The listing builds one solid part. Answer for the finished solid, in the listing's coordinates (mm). Face numbers are marked on the shaded views. A direction names the side the tool comes from. Give positions to 0.01 mm unless a question says otherwise; leave off trailing zeros. Order: outer loops, then holes, each group sorted by start corner. A loop starts at its lowest first (then second) coordinate and runs counter-clockwise, first axis right, second up. Notation, with made-up numbers: (69, 23.5) - (117, 23.5) arc R27 cw to (117, 51.5) - close; hole circle Ø5 at (28, 25). An arc over 180 degrees is marked (long way). Write each question's results on one line, items separated by ' | '. Start each with the question number.
1. Section D-D (x = -2.5) is taken. Give the vertices of the cut face in (y, z).
2. Find the intervals of material crossed by L1, parallel to Y at x = -10, z = 9; L2, parallel to Y at x = -9.25, z = 5.5; L3, parallel to X at y = -122.5, z = 1.25, in increasing order.
3. Determine the mould class of the marked faces 5, 6 and 7 for opening direction X: released by +X, released by -X, zero draft, split by the parting line, or undercut.
4. Flat-ended cylindrical pins translate along their axes: pin 1 (8 mm diameter, centred on y = -46, z = 5, fed in from +X); pin 2 (5 mm diameter, centred on x = -14.5, z = 6, fed in from +Y); pin 3 (4 mm diameter, centred on x = -10, y = -32.71, fed in from +Z); pin 4 (4 mm diameter, centred on x = -12, z = 8, fed in from -Y). Find the tip coordinate at first contact, or state that the pin passes through.
5. Which of the six approach directions +Z, -Z, +X, -X, +Y, -Y give full straight-line access (tool end or side, diameter ignored) to the marked faces 1, 2, 3 and 4?
6. Section C-C (z = 11) is taken. Give the vertices of the cut face in (x, y), and give its area (3 significant figures).
7. Section A-A (y = -123.5) is taken. Give the vertices of the cut face in (x, z).
8. Section B-B (x = -10) is taken. Give the vertices of the cut face in (y, z), and give its area (3 significant figures).
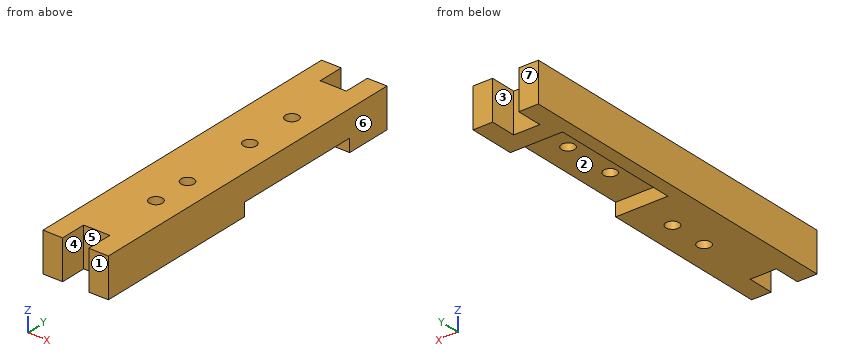
Autodesk Inventor part; units mm, degrees
ref_plane "YZ Plane" through (0, 0, 0) normal (1, 0, 0) x (0, 1, 0)
ref_plane "XZ Plane" through (0, 0, 0) normal (0, 1, 0) x (-1, 0, 0)
ref_plane "XY Plane" through (0, 0, 0) normal (0, 0, 1) x (1, 0, 0)
sketch "Sketch1" plane through (0, 0, 0) normal (0, 0, 1) x (1, 0, 0)
  circle A0 centre (-175, 0) radius 225 construction
  circle A1 centre (-175, 0) radius 200 construction
  line L0 (-25, 0) -> (-25, -132.2876)
  line L1 (-17.5, 0) -> (-17.5, -10)
  line L2 (-17.5, -10) -> (-7.5, -10)
  line L3 (-17.5, -10) -> (-7.5, -10) construction
  line L4 (-7.5, -10) -> (-7.5, 0)
  line L5 (-25, 0) -> (-17.5, 0)
  line L6 (-7.5, 0) -> (0, 0)
  line L7 (0, 0) -> (0, -132.2876)
  line L8 (-17.5, -132.2876) -> (-17.5, -122.2876)
  line L9 (-17.5, -132.2876) -> (-7.5, -132.2876) construction
  line L10 (-17.5, -122.2876) -> (-7.5, -122.2876)
  line L11 (-7.5, -122.2876) -> (-7.5, -132.2876)
  line L12 (-25, -132.2876) -> (-17.5, -132.2876)
  line L13 (-7.5, -132.2876) -> (0, -132.2876)
  dimension "d0" = 450
  dimension "d1" = 25
  dimension "d2" = 175
  dimension "d3" = 25
  dimension "d5" = 10
  dimension "d6" = 10
  dimension "d7" = 0
  dimension "d8" = 7.5
  dimension "d11" = 10
  dimension "d12" = 90
  dimension "d13" = 10
  dimension "d14" = 90
extrude "Extrusion1" add sketch "Sketch1" along normal blind 15
sketch "Sketch2" plane through (0, 0, 15) normal (0, 0, 1) x (1, 0, 0)
  line L0 (0, -17.7124) -> (-20, -17.7124) construction
  line L1 (-20, -17.7124) -> (-20, -67.7124) construction
  line L2 (-20, -67.7124) -> (0, -67.7124) construction
  line L3 (0, -67.7124) -> (0, -17.7124) construction
  line L4 (-7.5, -132.2876) -> (0, -132.2876) construction
  circle A0 centre (-10, -32.7124) radius 2.5
  circle A1 centre (-10, -52.7124) radius 2.5
  point P0 (0, 0)
  dimension "d15" = 20
  dimension "d16" = 50
  dimension "d17" = 64.5751
  dimension "d18" = 5
  dimension "d19" = 5
  dimension "d20" = 15
  dimension "d21" = 15
  dimension "d22" = 10
  dimension "d23" = 10
extrude "Extrusion2" cut sketch "Sketch2" against normal through all
thread "Thread1"
thread "Thread2"
sketch "Sketch3" plane through (0, 0, 15) normal (0, 0, 1) x (1, 0, 0)
  circle A0 centre (-10, -82.2876) radius 2.5
  circle A1 centre (-10, -97.2876) radius 2.5
  line L0 (0, -132.2876) -> (0, 0)
  line L1 (-7.5, -132.2876) -> (0, -132.2876)
  dimension "d30" = 5
  dimension "d31" = 5
  dimension "d32" = 10
  dimension "d33" = 10
  dimension "d34" = 15
  dimension "d35" = 35
extrude "Extrusion3" cut sketch "Sketch3" against normal through all
thread "Thread3"
thread "Thread4"
sketch "Sketch5" plane through (0, 0, 0) normal (0, 0, -1) x (-1, 0, 0)
  line L0 (0, -17.7124) -> (20, -17.7124)
  line L1 (20, -17.7124) -> (20, -67.7124)
  line L2 (20, -67.7124) -> (0, -67.7124)
  line L3 (0, -67.7124) -> (0, -17.7124)
  point P0 (0, 0)
  dimension "d50" = 20
  dimension "d51" = 50
  dimension "d52" = 17.7124
extrude "Extrusion5" cut sketch "Sketch5" against normal blind 5
properties part number "CP002" material "ABS Plastic"
Reported:
1) outline: (-132.29, 0) - (-67.71, 0) - (-67.71, 5) - (-17.71, 5) - (-17.71, 0) - (0, 0) - (0, 15) - (-132.29, 15) - close
2) L1: -122.29 to -99.79, -94.79 to -84.79, -79.79 to -55.21, -50.21 to -35.21, -30.21 to -10 | L2: -122.29 to -99.67, -94.9 to -84.67, -79.9 to -55.1, -50.33 to -35.1, -30.33 to -10 | L3: -25 to -17.5, -7.5 to 0
3) face 5: undercut | face 6: released by +X | face 7: zero draft
4) pin 1: x = 0 | pin 2: y = -10 | pin 3: through | pin 4: y = -122.29
5) face 1: +Z, -Z, +X, -X, -Y | face 2: -Z, +X | face 3: +Z, -Z, +Y | face 4: +Z, -Z, -Y
6) outline: (-25, -132.29) - (-17.5, -132.29) - (-17.5, -122.29) - (-7.5, -122.29) - (-7.5, -132.29) - (0, -132.29) - (0, 0) - (-7.5, 0) - (-7.5, -10) - (-17.5, -10) - (-17.5, 0) - (-25, 0) - close; hole circle Ø5 at (-10, -97.29); hole circle Ø5 at (-10, -82.29); hole circle Ø5 at (-10, -52.71); hole circle Ø5 at (-10, -32.71) | area: 3,030 mm²
7) outline: (-25, 0) - (-17.5, 0) - (-17.5, 15) - (-25, 15) - close; (-7.5, 0) - (0, 0) - (0, 15) - (-7.5, 15) - close
8) outline: (-122.29, 0) - (-99.79, 0) - (-99.79, 15) - (-122.29, 15) - close; (-94.79, 0) - (-84.79, 0) - (-84.79, 15) - (-94.79, 15) - close; (-79.79, 0) - (-67.71, 0) - (-67.71, 5) - (-55.21, 5) - (-55.21, 15) - (-79.79, 15) - close; (-50.21, 5) - (-35.21, 5) - (-35.21, 15) - (-50.21, 15) - close; (-30.21, 5) - (-17.71, 5) - (-17.71, 0) - (-10, 0) - (-10, 15) - (-30.21, 15) - close | area: 1,180 mm²
